The listing builds one solid part. Answer for the finished solid, in the listing's coordinates (mm). A direction names the side the tool comes from. Coordinates: 2 decimals unless noted, no trailing zeros. Write each loop counter-clockwise with the first axis right and the second up, starting at its lowest first coordinate (ties: lowest second). Pieces come first, ordered by that corner, then holes. Notation, with made-up numbers: M 80,-32.75 L 88,-32.75 A35 ccw 88,0.25 Z; hole C 10.5,54.25 d2. An arc over 180 degrees is marked long. Answer as CSV lines item,"result".
```python
from build123d import *

# Parameters (mm, degrees)
SKETCH1_W           = 14
SKETCH1_H           = 14
SKETCH1_R           = 1.6
BOSS_EXTRUDE1_DEPTH = 3
SKETCH2_R           = 1.6
BOSS_EXTRUDE2_DEPTH = 3
BOSS_EXTRUDE3_START = -4.5
BOSS_EXTRUDE3_DEPTH = 2.5


with BuildPart() as part:
    # Sketch1 → Boss-Extrude1 (new body)
    with BuildSketch(Plane(origin=(0, 0, 0), x_dir=(1, 0, 0), z_dir=(0, 1, 0))):
        Rectangle(SKETCH1_W, SKETCH1_H)
        with Locations(Location((0, 0, 0), (0, 0, 270))):
            Circle(SKETCH1_R, mode=Mode.SUBTRACT)
    extrude(amount=BOSS_EXTRUDE1_DEPTH)

    # Sketch2 → Boss-Extrude2 (add)
    with BuildSketch(Plane(origin=(0, 0, -7), x_dir=(-1, 0, 0), z_dir=(0, 0, -1))):
        Polygon((-7, 3), (-7, 0), (7, 0), (7, 3), (7, 17), (-7, 17), align=None)
        with Locations((0, 10)):
            Circle(SKETCH2_R, mode=Mode.SUBTRACT)
    extrude(amount=BOSS_EXTRUDE2_DEPTH)

    # Sketch5 → Boss-Extrude3 (add)
    with BuildSketch(Plane(origin=(0, 0, 0), x_dir=(0, 0, -1), z_dir=(1, 0, 0)).offset(BOSS_EXTRUDE3_START)):
        Polygon((7, 17), (5, 17), (-7, 5), (-7, 3), (7, 3), align=None)
    boss_extrude3 = extrude(amount=-BOSS_EXTRUDE3_DEPTH)

    # Mirror2: Boss-Extrude3 across plane
    add(boss_extrude3.mirror(Plane(origin=(0, 0, 0), x_dir=(0, 0, 1), z_dir=(1, 0, 0))))


solid = part.part
```
Q1. Straight lines are drawn through the part: line 1 (X direction, y = 12, z = -1.5); line 2 (X direction, y = 1.45, z = 0); line 3 (Y direction, x = -3.25, z = -5). For each, find the intervals that lie inside material, in ascending order.
Output:
line 1,"-7 to -4.5, 4.5 to 7"
line 2,"-7 to -1.6, 1.6 to 7"
line 3,"0 to 3"
Q2. Find section D-D (z = -7.5). Give the vertices of the cut face in (x, y), and give its area (3 significant figures).
Output:
outline,"M -7,0 L 7,0 L 7,17 L -7,17 Z; hole C 0,10 d3.2"
area,"230 mm2"
Q3. For faces 1 (the flat face through (6, 11, 1)), 2 (the flat face through (-4.5, 9, -1)), determine the directions among +Z, -Z, +X, -X, +Y, -Y from which every point of the face is accessible in a straight line to the end or side of a thin tool.
Output:
face 1,"+Z, +X, -X, +Y"
face 2,"+Z, +Y"
Q4. Find section A-A (z = 0). Give the vertices of the cut face in (x, y).
Output:
outline,"M -7,0 L -1.6,0 L -1.6,3 L -4.5,3 L -4.5,12 L -7,12 Z; M 1.6,0 L 7,0 L 7,12 L 4.5,12 L 4.5,3 L 1.6,3 Z"
Q5. Flat-ended cylindrical pins translate along their axes: pin 1 Ø2.5 at (x, y) = (-1.5, 11) entering from +Z; pin 2 Ø4.5 at (x, z) = (-2, 3.5) entering from +Y; pin 3 Ø3 at (x, z) = (0, 0) entering from +Y. Find the tip coordinate at first contact, or state that the pin passes through.
Output:
pin 1,"z = -7"
pin 2,"y = 3"
pin 3,"through"
Q6. Find section C-C (y = 9.5). Give the vertices of the cut face in (x, z).
Output:
outline,"M -7,-10 L -1.52,-10 L -1.52,-7 L -4.5,-7 L -4.5,2.5 L -7,2.5 Z; M 1.52,-10 L 7,-10 L 7,2.5 L 4.5,2.5 L 4.5,-7 L 1.52,-7 Z"
Q7. The mould has two halves that part along Z. Classify faces 3 (the cylindrical face through (-0.97, 1.48, -1.27)), 4 (the flat face through (0, 12, -7)), 5 (the flat face through (2, 9, -10)), 6 (the cylindrical face through (0.35, 8.44, -8.48)): pulls with the +Z half, pulls with the -Z half, needs draft (parallel to the pull), parting line crosses it, or undercut.
Output:
face 3,"undercut"
face 4,"pulls with the +Z half"
face 5,"pulls with the -Z half"
face 6,"needs draft"
Q8. Find section B-B (x = 0). Give the vertices of the cut face in (y, z).
Output:
outline,"M 0,-10 L 8.4,-10 L 8.4,-7 L 3,-7 L 3,-1.6 L 0,-1.6 Z; M 0,1.6 L 3,1.6 L 3,7 L 0,7 Z; M 11.6,-10 L 17,-10 L 17,-7 L 11.6,-7 Z"
